Geometry: final body of the model. Coordinates: model frame, mm. Coordinates: 2 decimals unless noted, no trailing zeros. Write each loop counter-clockwise with the first axis right and the second up, starting at its lowest first coordinate (ties: lowest second). Pieces come first, ordered by that corner, then holes. Notation, with made-up numbers: (-25.5, 56) - (30.5, 56) arc R3 ccw to (30.5, 60) - close; hole circle Ø10 at (-28.75, 54.5). An arc over 180 degrees is marked (long way). Answer as a JSON object with one key per item and string values. Group by question number.
Item 1: Section D-D on y = 2.1. State how many separate pieces and enclosed holes the cut face has, and give its area (3 significant figures).
Item 2: Section C-C on x = 16. Return loops of the section in (y, z).
Item 3: Section B-B on x = 39. Return loops of the section in (y, z), and give its area (3 significant figures).
Item 4: First-contact query: pin 1 Ø0.9 at (x, y) = (63, 2) entering from -Z; pin 2 Ø1 at (x, y) = (49.5, 1) entering from -Z; pin 3 Ø0.9 at (x, y) = (-38, 2) entering from +Z. Flat tips, straight axial feed; report the tip coordinate or a pass-through.
Item 5: Section A-A on x = 0. Return loops of the section in (y, z).
Item 6: Line query: line 1 along X through (y, z) = (1.3, 21); line 2 along X through (y, z) = (1.9, -18.5); line 3 along Z through (x, y) = (-7.5, 1.3). Output: solid intervals per line, ascending. Write a range as from..to.
```python
from build123d import *

# Parameters (mm, degrees)
SKETCH2_R            = 29
SKETCH2_R_2          = 23.5
BOSS_EXTRUDE1_DEPTH  = 3
SKETCH2_3_R          = 1
BOSS_EXTRUDE2_DEPTH  = 3
FILLET1_R            = 5
SKETCH3_R            = 1
CUT_EXTRUDE1_DEPTH   = 3
CIRPATTERN1_COUNT    = 3
FILLET1_OF_MIRROR1_R = 5


with BuildPart() as part:
    # Sketch2 → Boss-Extrude1 (new body)
    with BuildSketch(Plane(origin=(0, 0, 0), x_dir=(1, 0, 0), z_dir=(0, 1, 0))):
        with Locations(Location((0, 0, 0), (0, 0, 270))):
            Circle(SKETCH2_R)
        with Locations(Location((0, 0, 0), (0, 0, 270))):
            Circle(SKETCH2_R_2, mode=Mode.SUBTRACT)
    extrude(amount=BOSS_EXTRUDE1_DEPTH)

    # Sketch2<3> → Boss-Extrude2 (add)
    with BuildSketch(Plane(origin=(0, 0, 0), x_dir=(1, 0, 0), z_dir=(0, 1, 0))):
        with BuildLine():
            Line((44.819347292, 15), (24.819347292, 15))
            ThreePointArc((24.819347292, 15), (27.935291939, 7.78585026), (29, 0))
            ThreePointArc((29, 0), (27.935291939, -7.78585026), (24.819347292, -15))
            Line((24.819347292, -15), (44.819347292, -15))
            Line((44.819347292, -15), (52.319347292, -22.5))
            Line((52.319347292, -22.5), (66.319347292, -22.5))
            Line((66.319347292, -22.5), (66.319347292, 22.5))
            Line((66.319347292, 22.5), (52.319347292, 22.5))
            Line((52.319347292, 22.5), (44.819347292, 15))
        make_face()
        with Locations(Location((62.319347292, -10, 0), (0, 0, 270))):
            Circle(SKETCH2_3_R, mode=Mode.SUBTRACT)
        with Locations(Location((62.319347292, 10, 0), (0, 0, 270))):
            Circle(SKETCH2_3_R, mode=Mode.SUBTRACT)
    boss_extrude2 = extrude(amount=BOSS_EXTRUDE2_DEPTH)

    # Fillet1
    fillet1_edges = [part.edges().sort_by_distance(p)[0] for p in [
        (44.819347292, 1.5, -15),
        (52.319347292, 1.5, -22.5),
        (52.319347292, 1.5, 22.5),
        (44.819347292, 1.5, 15),
        (24.819347292, 1.5, 15),
        (24.819347292, 1.5, -15),
    ]]
    fillet(fillet1_edges, radius=FILLET1_R)

    # Sketch3 → Cut-Extrude1 (cut)
    with BuildSketch(Plane(origin=(0, 3, 0), x_dir=(1, 0, 0), z_dir=(0, 1, 0))):
        with Locations(Location((13.25, 22.9496732, 0), (0, 0, 270))):
            Circle(SKETCH3_R)
    cut_extrude1 = extrude(amount=-CUT_EXTRUDE1_DEPTH, mode=Mode.SUBTRACT)

    # CirPattern1: Cut-Extrude1 ×3 about axis
    cirpattern1_axis = Axis((0, 0, 0), (0, 1, 0))
    for i in range(1, CIRPATTERN1_COUNT):
        add(cut_extrude1.rotate(cirpattern1_axis, i * 360 / CIRPATTERN1_COUNT), mode=Mode.SUBTRACT)

    # Mirror1: Boss-Extrude2 across plane
    add(boss_extrude2.mirror(Plane(origin=(0, 0, 0), x_dir=(0, 0, 1), z_dir=(1, 0, 0))))

    # Fillet1 of Mirror1
    fillet1_of_mirror1_edges = [part.edges().sort_by_distance(p)[0] for p in [
        (-44.819347292, 1.5, -15),
        (-52.319347292, 1.5, -22.5),
        (-52.319347292, 1.5, 22.5),
        (-44.819347292, 1.5, 15),
        (-24.819347292, 1.5, 15),
        (-24.819347292, 1.5, -15),
    ]]
    fillet(fillet1_of_mirror1_edges, radius=FILLET1_OF_MIRROR1_R)


solid = part.part
```
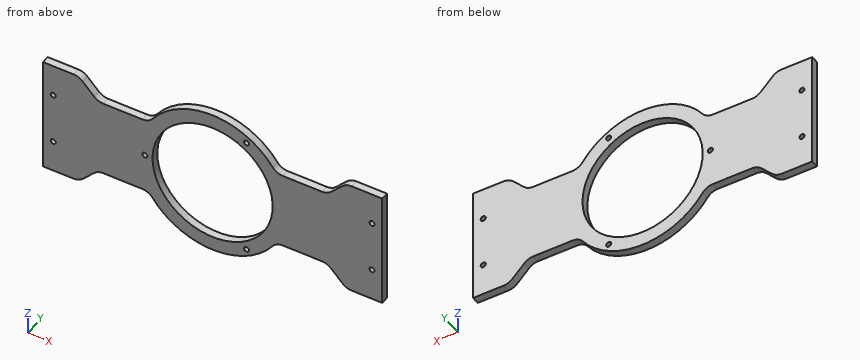
Checks:
{
 "1": {"separate pieces": "1", "enclosed holes": "8", "area": "3,740 mm^2"},
 "2": {"outline": "(0, -24.19) - (3, -24.19) - (3, -17.21) - (0, -17.21) - close; (0, 17.21) - (3, 17.21) - (3, 24.19) - (0, 24.19) - close"},
 "3": {"outline": "(0, -15) - (3, -15) - (3, 15) - (0, 15) - close", "area": "90.0 mm^2"},
 "4": {"pin 1": "z = -22.5", "pin 2": "z = -20.18", "pin 3": "z = 15"},
 "5": {"outline": "(0, -29) - (3, -29) - (3, -23.5) - (0, -23.5) - close; (0, 23.5) - (3, 23.5) - (3, 29) - (0, 29) - close"},
 "6": {"line 1": "-66.32..-50.82, -20..-10.55, 10.55..20, 50.82..66.32", "line 2": "-66.32..-48.32, -22.33..-14.49, 14.49..22.33, 48.32..66.32", "line 3": "-28.01..-22.27, 22.27..28.01"}
}
